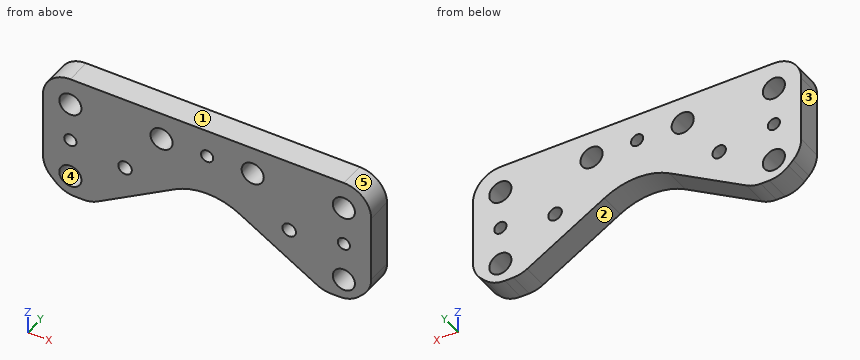
```python
from build123d import *

# Parameters (mm, degrees)
SKETCH1_R           = 15
BOSS_EXTRUDE1_DEPTH = 6
SKETCH2_R           = 1.5
CUT_EXTRUDE1_DEPTH  = 92.777339251
CUT_EXTRUDE2_DEPTH  = 92.777339251
SKETCH13_R          = 1.65
M4_TAP_DEPTH        = 85.985660555
SKETCH15_R          = 2.65
M5_THROUGH_DEPTH    = 83.615146916
FILLET1_R           = 6.35
CUT_EXTRUDE4_START  = -10
CUT_EXTRUDE4_DEPTH  = 10
FILLET2_R           = 6.35
SKETCH17_R          = 1.5
CUT_EXTRUDE5_DEPTH  = 82.827930172
MOVE_FACE1_BY       = 0.08
MOVE_FACE1_2_BY     = 0.08
MOVE_FACE1_3_BY     = 0.08
MOVE_FACE1_4_BY     = 0.08
MOVE_FACE1_5_BY     = 0.08
MOVE_FACE1_6_BY     = 0.08
MOVE_FACE1_7_BY     = 0.08
MOVE_FACE1_8_BY     = 0.08
MOVE_FACE1_9_BY     = 0.08
MOVE_FACE1_10_BY    = 0.08
MOVE_FACE1_11_BY    = 0.08


with BuildPart() as part:
    # Sketch1 → Boss-Extrude1 (new body)
    with BuildSketch(Plane(origin=(0, 0, 0), x_dir=(1, 0, 0), z_dir=(0, 1, 0))):
        Polygon((0, 0), (76.2, 0), (76.2, 50.8), (38.1, 50.8), (0, 50.8), align=None)
        with Locations(Location((38.1, 30.8, 0), (0, 0, 270))):
            Circle(SKETCH1_R, mode=Mode.SUBTRACT)
    extrude(amount=BOSS_EXTRUDE1_DEPTH)

    # Sketch2 → Cut-Extrude1 (cut, through all)
    with BuildSketch(Plane(origin=(0, 6, 0), x_dir=(1, 0, 0), z_dir=(0, 1, 0))):
        with Locations(Location((19.05, 30.8, 0), (0, 0, 270))):
            Circle(SKETCH2_R)
        with Locations(Location((57.15, 30.8, 0), (0, 0, 90))):
            Circle(SKETCH2_R)
    extrude(amount=-CUT_EXTRUDE1_DEPTH, mode=Mode.SUBTRACT)

    # Sketch9 → Cut-Extrude2 (cut, through all)
    with BuildSketch(Plane(origin=(0, 6, 0), x_dir=(1, 0, 0), z_dir=(0, 1, 0))):
        with BuildLine():
            Line((0, 50.8), (76.2, 50.8))
            Line((76.2, 50.8), (76.2, 24.45))
            Line((76.2, 24.45), (63.5, 37.15))
            Line((63.5, 37.15), (53.1, 37.15))
            Line((53.1, 37.15), (53.1, 30.8))
            ThreePointArc((53.1, 30.8), (38.1, 15.8), (23.1, 30.8))
            Line((23.1, 30.8), (23.1, 37.15))
            Line((23.1, 37.15), (12.7, 37.15))
            Line((12.7, 37.15), (0, 24.45))
            Line((0, 24.45), (0, 50.8))
        make_face()
    extrude(amount=-CUT_EXTRUDE2_DEPTH, mode=Mode.SUBTRACT)

    # Sketch13 → M4-tap (cut, through all)
    with BuildSketch(Plane(origin=(0, 6, 0), x_dir=(1, 0, 0), z_dir=(0, 1, 0))):
        with Locations(Location((19.05, 17.15, 0), (0, 0, 270))):
            Circle(SKETCH13_R)
        with Locations(Location((57.15, 17.15, 0), (0, 0, 270))):
            Circle(SKETCH13_R)
    extrude(amount=-M4_TAP_DEPTH, mode=Mode.SUBTRACT)

    # Sketch15 → M5-through (cut, through all)
    with BuildSketch(Plane(origin=(0, 6, -5.8), x_dir=(1, 0, 0), z_dir=(0, -1, 0))):
        with Locations(Location((6.35, -18.65, 0), (0, 0, 270))):
            Circle(SKETCH15_R)
        with Locations(Location((6.35, -0.55, 0), (0, 0, 270))):
            Circle(SKETCH15_R)
        with Locations(Location((27.516666667, -0.55, 0), (0, 0, 270))):
            Circle(SKETCH15_R)
        with Locations(Location((48.683333333, -0.55, 0), (0, 0, 270))):
            Circle(SKETCH15_R)
        with Locations(Location((69.85, -0.55, 0), (0, 0, 270))):
            Circle(SKETCH15_R)
        with Locations(Location((69.85, -18.65, 0), (0, 0, 270))):
            Circle(SKETCH15_R)
    extrude(amount=M5_THROUGH_DEPTH, mode=Mode.SUBTRACT)

    # Fillet1
    fillet1_edges = [part.edges().sort_by_distance(p)[0] for p in [
        (76.2, 3, 0),
        (0, 3, 0),
        (0, 3, -24.45),
        (76.2, 3, -24.45),
        (63.5, 3, -37.15),
        (53.1, 3, -37.15),
        (23.1, 3, -37.15),
        (12.7, 3, -37.15),
    ]]
    fillet(fillet1_edges, radius=FILLET1_R - 0.0001)  # a hair under: the kernel refuses the full size

    # Sketch16 → Cut-Extrude4 (cut)
    with BuildSketch(Plane(origin=(0, 6, 0), x_dir=(1, 0, 0), z_dir=(0, 1, 0)).offset(CUT_EXTRUDE4_START)):
        with BuildLine():
            Line((30.524360743, 17.853583899), (11.1125, 29.2125))
            Line((11.1125, 29.2125), (4.7625, 29.2125))
            Line((4.7625, 29.2125), (38.1, 62.55))
            Line((38.1, 62.55), (71.4375, 29.2125))
            Line((71.4375, 29.2125), (65.0875, 29.2125))
            Line((65.0875, 29.2125), (45.675639257, 17.853583899))
            ThreePointArc((45.675639257, 17.853583899), (38.1, 15.8), (30.524360743, 17.853583899))
        make_face()
    extrude(amount=CUT_EXTRUDE4_DEPTH, mode=Mode.SUBTRACT)

    # Fillet2
    fillet2_edges = [part.edges().sort_by_distance(p)[0] for p in [
        (11.1125, 3, -29.2125),
        (4.7625, 3, -29.2125),
        (71.4375, 3, -29.2125),
        (65.0875, 3, -29.2125),
    ]]
    fillet(fillet2_edges, radius=FILLET2_R)

    # Sketch17 → Cut-Extrude5 (cut, through all)
    with BuildSketch(Plane(origin=(0, 6, 0), x_dir=(-1, 0, 0), z_dir=(0, 1, 0))):
        with Locations(Location((-6.35, -15.4, 0), (0, 0, 90))):
            Circle(SKETCH17_R)
        with Locations(Location((-38.1, -6.35, 0), (0, 0, 90))):
            Circle(SKETCH17_R)
        with Locations(Location((-69.85, -15.4, 0), (0, 0, 90))):
            Circle(SKETCH17_R)
    extrude(amount=-CUT_EXTRUDE5_DEPTH, mode=Mode.SUBTRACT)

    # Move Face1: a curved face moved outward by 0.08
    add(Solid.thicken(part.faces().sort_by_distance((6.35, 3, -21.8))[0], MOVE_FACE1_BY))

    # Move Face1 2: a curved face moved outward by 0.08
    add(Solid.thicken(part.faces().sort_by_distance((19.05, 3, -18.8))[0], MOVE_FACE1_2_BY))

    # Move Face1 3: a curved face moved outward by 0.08
    add(Solid.thicken(part.faces().sort_by_distance((57.15, 3, -18.8))[0], MOVE_FACE1_3_BY))

    # Move Face1 4: a curved face moved outward by 0.08
    add(Solid.thicken(part.faces().sort_by_distance((6.35, 3, -3.7))[0], MOVE_FACE1_4_BY))

    # Move Face1 5: a curved face moved outward by 0.08
    add(Solid.thicken(part.faces().sort_by_distance((27.516666667, 3, -3.7))[0], MOVE_FACE1_5_BY))

    # Move Face1 6: a curved face moved outward by 0.08
    add(Solid.thicken(part.faces().sort_by_distance((48.683333333, 3, -3.7))[0], MOVE_FACE1_6_BY))

    # Move Face1 7: a curved face moved outward by 0.08
    add(Solid.thicken(part.faces().sort_by_distance((69.85, 3, -3.7))[0], MOVE_FACE1_7_BY))

    # Move Face1 8: a curved face moved outward by 0.08
    add(Solid.thicken(part.faces().sort_by_distance((69.85, 3, -21.8))[0], MOVE_FACE1_8_BY))

    # Move Face1 9: a curved face moved outward by 0.08
    add(Solid.thicken(part.faces().sort_by_distance((6.35, 3, -16.9))[0], MOVE_FACE1_9_BY))

    # Move Face1 10: a curved face moved outward by 0.08
    add(Solid.thicken(part.faces().sort_by_distance((38.1, 3, -7.85))[0], MOVE_FACE1_10_BY))

    # Move Face1 11: a curved face moved outward by 0.08
    add(Solid.thicken(part.faces().sort_by_distance((69.85, 3, -16.9))[0], MOVE_FACE1_11_BY))


solid = part.part
```
Build history of the part. All positions in model axes, mm. Face numbers are marked on the shaded views. A direction names the side the tool comes from. Round coordinates to 2 decimals unless told otherwise and drop trailing zeros. Write each loop counter-clockwise with the first axis right and the second up, starting at its lowest first coordinate (ties: lowest second). Pieces come first, ordered by that corner, then holes. Notation, with made-up numbers: (-19.5, -13.75) -> (37.5, -13.75) arc R31 ccw to (37.5, 24.25) -> close; hole circle Ø1 at (55, 33). An arc over 180 degrees is marked (long way). Put each result on its own line as item: value.
Item 1: Flat gauge pin, fed straight in: P1, Ø3, axis at x = 69.85, z = -6.35, coming from the -Y side. Where does the tip first touch, or does it go through?
Here are the results:
P1: passes through
Item 2: Slice it at A-A, the plane x = 58. Give the cut face in (y, z), plus the area to 3 significant figures.
Here are the results:
outline: (0, -25.07) -> (6, -25.07) -> (6, -18.47) -> (0, -18.47) -> close; (0, -15.83) -> (6, -15.83) -> (6, 0) -> (0, 0) -> close
area: 135 mm^2
Item 3: Two-plate mould, pull along Z, no slides. Class the marked faces 3, 4 and 5: pulls with the +Z half, pulls with the -Z half, needs draft (parallel to the pull), parting line crosses it, or undercut.
Here are the results:
face 3: needs draft
face 4: undercut
face 5: pulls with the +Z half
Item 4: Slice it at B-B, the plane z = -23.5. Give the cut face in (x, y), plus the area to 3 significant figures.
Here are the results:
outline: (0.23, 0) -> (3.96, 0) -> (3.96, 6) -> (0.23, 6) -> close; (8.74, 0) -> (20.87, 0) -> (20.87, 6) -> (8.74, 6) -> close; (55.33, 0) -> (67.46, 0) -> (67.46, 6) -> (55.33, 6) -> close; (72.24, 0) -> (75.97, 0) -> (75.97, 6) -> (72.24, 6) -> close
area: 190 mm^2
Item 5: Tool access for the marked faces 1 and 2: list every direction of +Z, -Z, +X, -X, +Y, -Y with a clear straight run to the whole face (end or side of a thin tool).
Here are the results:
face 1: +Z, +X, -X, +Y, -Y
face 2: -Z, +Y, -Y
Item 6: Slice it at D-D, the plane x = 19.05. Give the cut face in (y, z), plus the area to 3 significant figures.
Here are the results:
outline: (0, -24.57) -> (6, -24.57) -> (6, -18.72) -> (0, -18.72) -> close; (0, -15.58) -> (6, -15.58) -> (6, 0) -> (0, 0) -> close
area: 129 mm^2
Item 7: Wall check: probe 1 along X at (y, z) = (1.4, -6.35); probe 2 along X at (y, z) = (4.5, -26.5); probe 3 along X at (y, z) = (4.5, -23.75). Give the ranges that are in metal, low to high. Write a range as from..to.
Here are the results:
probe 1: x = 0..3.78, 8.92..24.95, 30.09..36.68, 39.52..46.11, 51.25..67.28, 72.42..76.2
probe 2: x = 2.05..4.8, 7.9..15.75, 60.45..68.3, 71.4..74.15
probe 3: x = 0.3..3.88, 8.82..20.45, 55.75..67.38, 72.32..75.9
Item 8: Slice it at C-C, the plane y = 4.5. Count the separate pieces of the cut face and the enclosed holes in it, plus the area to 3 significant figures.
Here are the results:
separate pieces: 1
enclosed holes: 11
area: 1,610 mm^2
